Build history of the part. All positions in model axes, mm. Face numbers are marked on the shaded views. Give positions to 0.01 mm unless a question says otherwise; leave off trailing zeros. Write each loop counter-clockwise with the first axis right and the second up, starting at its lowest first coordinate (ties: lowest second). Pieces come first, ordered by that corner, then holes. Notation, with made-up numbers: (-23, -19) -> (21, -19) arc R7 cw to (21, -11) -> close; hole circle Ø3 at (86.5, 59.5). An arc over 180 degrees is marked (long way). One line per question, with ' | ' between items. Start each with the question number.
(1) Band-saw the part on B-B, the plane z = 45. Give the cut face in (x, y).
(2) Band-saw the part on A-A, the plane x = -102. Give the cut face in (y, z), and give its area (3 significant figures).
(3) Pull direction X, two halves, no side cores. Call the marked faces 1 and 2: released by +X, released by -X, zero draft, split by the parting line, or undercut.
(4) Band-saw the part on C-C, the plane y = 0.5. Count the separate pieces of the cut face and the enclosed holes in it, and give its area (3 significant figures).
(5) Pin check, flat tips, straight feed: P1, Ø4.5, axis at x = 38.86, z = 56.13, coming from the +Y side; P2, Ø12, axis at x = 25.5, z = 21.5, coming from the +Y side. Stop position of each tip, or through.
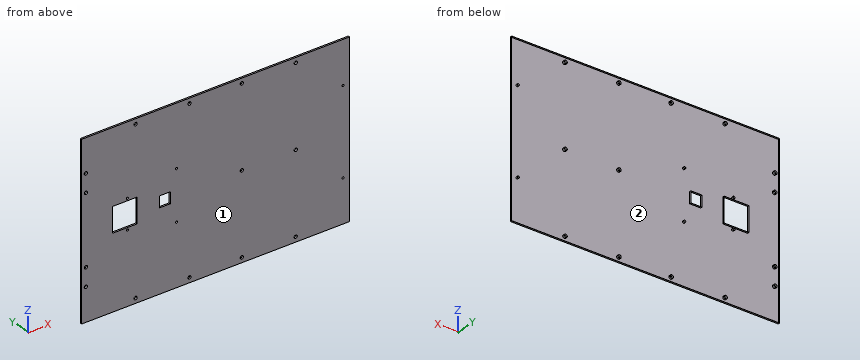
from build123d import *

# Parameters (mm, degrees)
SKETCH1_W                    = 199.39
SKETCH1_H                    = 127
BOSS_EXTRUDE1_DEPTH          = 2.54
F_11_0_191_DIAMETER_HOLE1_D  = 4.8514
F_11_0_191_DIAMETER_HOLE2_D  = 4.8514
SKETCH8_W                    = 36.83
SKETCH8_H                    = 18.415
SKETCH8_W_2                  = 16.51
SKETCH8_H_2                  = 8.255
CUT_EXTRUDE1_DEPTH           = 2.54
F_11_0_191_DIAMETER_HOLE3_D  = 4.8514
F_31_0_12_DIAMETER_HOLE2_D   = 3.048
F_31_0_12_DIAMETER_HOLE3_D   = 3.048
F_1_8_0_125_DIAMETER_HOLE1_D = 3.048
SHELL1_T                     = -0.1016


with BuildPart() as part:
    # Sketch1 → Boss-Extrude1 (new body)
    with BuildSketch(Plane(origin=(0, 0, 0), x_dir=(1, 0, 0), z_dir=(0, 1, 0))):
        with Locations((-99.695, 0)):
            Rectangle(SKETCH1_W, SKETCH1_H)
        with Locations((99.695, 0)):
            Rectangle(SKETCH1_W, SKETCH1_H)
    boss_extrude1 = extrude(amount=BOSS_EXTRUDE1_DEPTH)

    # #11 (0.191) Diameter Hole1 (through all)
    with Locations(Plane(origin=(0, 2.54, 0), x_dir=(1, 0, 0), z_dir=(0, 1, 0))):
        with Locations((-193.167, -14.4018), (-193.04, 12.3444)):
            f_11_0_191_diameter_hole1 = Hole(F_11_0_191_DIAMETER_HOLE1_D / 2)

    # #11 (0.191) Diameter Hole2 (through all)
    with Locations(Plane(origin=(0, 2.54, 0), x_dir=(1, 0, 0), z_dir=(0, 1, 0))):
        with Locations((-119.126, -56.127777467), (-38.862, -56.127777467), (38.862, -56.127777467), (119.126, -56.127777467)):
            f_11_0_191_diameter_hole2 = Hole(F_11_0_191_DIAMETER_HOLE2_D / 2)

    # Sketch8 → Cut-Extrude1 (cut)
    with BuildSketch(Plane(origin=(0, 2.54, 0), x_dir=(1, 0, 0), z_dir=(0, 1, 0))):
        with Locations((-135.255, 54.2925)):
            Rectangle(SKETCH8_W, SKETCH8_H)
        with Locations((-75.565, 59.3725)):
            Rectangle(SKETCH8_W_2, SKETCH8_H_2)
    cut_extrude1 = extrude(amount=-CUT_EXTRUDE1_DEPTH, mode=Mode.SUBTRACT)

    # Mirror6: Boss-Extrude1, #11 (0.191) Diameter Hole1, #11 (0.191) Diameter Hole2, Cut-Extrude1 across plane
    add(boss_extrude1.mirror(Plane(origin=(0, 2.54, -63.5), x_dir=(1, 0, 0), z_dir=(0, 0, -1))))
    add(f_11_0_191_diameter_hole1.mirror(Plane(origin=(0, 2.54, -63.5), x_dir=(1, 0, 0), z_dir=(0, 0, -1))), mode=Mode.SUBTRACT)
    add(f_11_0_191_diameter_hole2.mirror(Plane(origin=(0, 2.54, -63.5), x_dir=(1, 0, 0), z_dir=(0, 0, -1))), mode=Mode.SUBTRACT)
    add(cut_extrude1.mirror(Plane(origin=(0, 2.54, -63.5), x_dir=(1, 0, 0), z_dir=(0, 0, -1))), mode=Mode.SUBTRACT)

    # #11 (0.191) Diameter Hole3 (through all)
    with Locations(Plane(origin=(0, 2.54, 0), x_dir=(1, 0, 0), z_dir=(0, 1, 0))):
        with Locations((119.126, 63.5), (38.862, 63.5)):
            Hole(F_11_0_191_DIAMETER_HOLE3_D / 2)

    # #31 (0.12) Diameter Hole2 (through all)
    with Locations(Plane(origin=(0, 2.54, 0), x_dir=(1, 0, 0), z_dir=(0, 1, 0))):
        with Locations((-131.318, 41.656), (-131.318, 85.344)):
            Hole(F_31_0_12_DIAMETER_HOLE2_D / 2)

    # #31 (0.12) Diameter Hole3 (through all)
    with Locations(Plane(origin=(0, 2.54, 0), x_dir=(1, 0, 0), z_dir=(0, 1, 0))):
        with Locations((-58.166, 100.33), (-58.166, 26.67)):
            Hole(F_31_0_12_DIAMETER_HOLE3_D / 2)

    # 1/8 (0.125) Diameter Hole1 (through all)
    with Locations(Plane(origin=(0, 2.54, 0), x_dir=(1, 0, 0), z_dir=(0, 1, 0))):
        with Locations((189.484, 0), (189.484, 127)):
            Hole(F_1_8_0_125_DIAMETER_HOLE1_D / 2)

    # Shell1
    shell1_openings = [part.faces().sort_by_distance(p)[0] for p in [
        (189.484, 2.54, 1.524),
    ]]
    offset(amount=SHELL1_T, openings=shell1_openings, kind=Kind.INTERSECTION)


solid = part.part
Results:
1) outline: (-199.39, 0) -> (199.39, 0) -> (199.39, 2.54) -> (199.29, 2.54) -> (199.29, 0.1) -> (-199.29, 0.1) -> (-199.29, 2.54) -> (-199.39, 2.54) -> close
2) outline: (0, -190.5) -> (2.54, -190.5) -> (2.54, -190.4) -> (0.1, -190.4) -> (0.1, 63.4) -> (2.54, 63.4) -> (2.54, 63.5) -> (0, 63.5) -> close | area: 26.3 mm²
3) face 1: zero draft | face 2: undercut
4) separate pieces: 23 | enclosed holes: 23 | area: 183 mm²
5) P1: passes through | P2: stops at y = 0.1
